For this review, take the finished solid that the model builds, in its own axes (mm). Coordinates: 2 decimals unless noted, no trailing zeros. Loops run counter-clockwise (first coordinate to the right, second up) from the corner with the lowest first, then second, coordinate; pieces in that order, holes last. Notation, with made-up numbers: (-4, 14) - (49, 14) arc R24 ccw to (49, 45) - close; hole circle Ø3 at (75, 9.5). An arc over 180 degrees is marked (long way). Use one line per item in the form item = value. Start each with the question number.
1. Add section B-B on x = 28.5. Give the boundary of the cut face in (y, z).
2. To check wall thickness, follow probe 1 along Y at (x, z) = (10, 3); probe 2 along X at (y, z) = (17.5, 4.5); probe 3 along Y at (x, z) = (28.5, 8). State the ranges of each line that lie inside material, in increasing order.
3. Add section A-A on x = -10. Give the boundary of the cut face in (y, z), and give its area (3 significant figures).
4. For pin 1 Ø5 at (x, y) = (3.5, -33.5) entering from -Z; pin 2 Ø2 at (x, y) = (-10, 18) entering from -Z (3 decimals), all flat-tipped, find the tip position at first contact; note any pin that passes through.
5. Add section C-C on z = 8.75. Give the boundary of the cut face in (x, y), and give its area (3 significant figures).
6. Add section D-D on y = 7. Give the boundary of the cut face in (x, z).
```python
from build123d import *

# Parameters (mm, degrees)
SKETCH_W        = 70
SKETCH_H        = 100
PAD_DEPTH       = 10
SKETCH001_R     = 3.25
POCKET_DEPTH    = 10.001
SKETCH002_R     = 1.7
POCKET001_DEPTH = 10.001
FILLET_R        = 5


with BuildPart() as part:
    # Sketch → Pad (new body)
    with BuildSketch(Plane.XY):
        Rectangle(SKETCH_W, SKETCH_H)
    extrude(amount=PAD_DEPTH)

    # Sketch001 (on Face6 of Pad) → Pocket (cut, through all)
    with BuildSketch(Plane.XY.offset(10)):
        with Locations((-27, 5)):
            Circle(SKETCH001_R)
        with Locations((28.5, 7)):
            Circle(SKETCH001_R)
    extrude(amount=-POCKET_DEPTH, mode=Mode.SUBTRACT)

    # Sketch002 (on Face5 of Pocket) → Pocket001 (cut, through all)
    with BuildSketch(Plane.XY.offset(10)):
        with Locations((-10, 18)):
            Circle(SKETCH002_R)
        with Locations((10, 18)):
            Circle(SKETCH002_R)
        with Locations((10, -18)):
            Circle(SKETCH002_R)
        with Locations((-10, -18)):
            Circle(SKETCH002_R)
    extrude(amount=-POCKET001_DEPTH, mode=Mode.SUBTRACT)

    # Fillet
    fillet_edges = [part.edges().sort_by_distance(p)[0] for p in [
        (35, -50, 5),
        (-35, -50, 5),
        (35, 50, 5),
        (-35, 50, 5),
    ]]
    fillet(fillet_edges, radius=FILLET_R)


solid = part.part
```
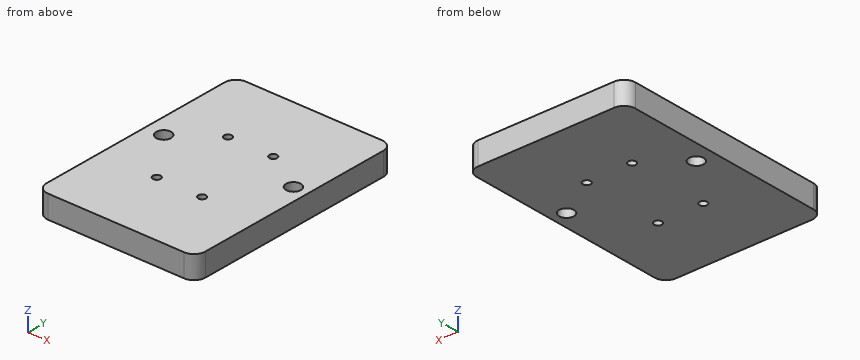
Conclusion:
q1.outline = (-50, 0) - (3.75, 0) - (3.75, 10) - (-50, 10) - close; (10.25, 0) - (50, 0) - (50, 10) - (10.25, 10) - close
q2.probe_1 = -50 to -19.7, -16.3 to 16.3, 19.7 to 50
q2.probe_2 = -35 to -11.62, -8.38 to 8.38, 11.62 to 35
q2.probe_3 = -50 to 3.75, 10.25 to 50
q3.outline = (-50, 0) - (-19.7, 0) - (-19.7, 10) - (-50, 10) - close; (-16.3, 0) - (16.3, 0) - (16.3, 10) - (-16.3, 10) - close; (19.7, 0) - (50, 0) - (50, 10) - (19.7, 10) - close
q3.area = 932 mm^2
q4.pin_1 = 0
q4.pin_2 = through
q5.outline = (-35, -45) arc R5 ccw to (-30, -50) - (30, -50) arc R5 ccw to (35, -45) - (35, 45) arc R5 ccw to (30, 50) - (-30, 50) arc R5 ccw to (-35, 45) - close; hole circle Ø6.5 at (-27, 5); hole circle Ø3.4 at (-10, -18); hole circle Ø3.4 at (-10, 18); hole circle Ø3.4 at (10, -18); hole circle Ø3.4 at (10, 18); hole circle Ø6.5 at (28.5, 7)
q5.area = 6,880 mm^2
q6.outline = (-35, 0) - (-29.56, 0) - (-29.56, 10) - (-35, 10) - close; (-24.44, 0) - (25.25, 0) - (25.25, 10) - (-24.44, 10) - close; (31.75, 0) - (35, 0) - (35, 10) - (31.75, 10) - close
